Autodesk Inventor part; units mm, degrees
ref_plane "Work Plane1" through (0, 0, 0) normal (0, 0, 1) x (1, 0, 0)
ref_plane "Work Plane2" through (-10.1976, -10.1976, 2) normal (0, 0, 1) x (0.910504, -0.4135003, 0)
ref_plane "YZ Plane" through (0, 0, 0) normal (1, 0, 0) x (0, 1, 0)
ref_plane "Work Plane1" through (0, 0, 0) normal (0, 0, 1) x (1, 0, 0)
sketch "Sketch1" plane through (0, 0, 0) normal (0, 0, 1) x (1, 0, 0)
  circle A0 centre (0, 0) radius 12.5
  circle A1 centre (0, -18) radius 2
  circle A2 centre (0, 18) radius 2
  circle A3 centre (-18, 0) radius 2
  circle A4 centre (18, 0) radius 2
  circle A5 centre (11.3137, 11.3137) radius 1.6
  circle A6 centre (-11.3137, -11.3137) radius 1.6
  circle A7 centre (-11.3137, 11.3137) radius 1.6
  circle A8 centre (11.3137, -11.3137) radius 1.6
  circle A9 centre (0, 0) radius 20.7
  circle A10 centre (-11.3137, 11.3137) radius 1.2295
  circle A11 centre (0, 18) radius 1.621
  circle A12 centre (11.3137, 11.3137) radius 1.2295
  circle A13 centre (18, 0) radius 1.621
  circle A14 centre (11.3137, -11.3137) radius 1.2295
  circle A15 centre (-11.3137, -11.3137) radius 1.2295
  circle A16 centre (0, -18) radius 1.621
  circle A17 centre (-18, 0) radius 1.621
ref_plane "Work Plane2" through (-10.1976, -10.1976, 2) normal (0, 0, 1) x (0.910504, -0.4135003, 0)
extrude "Extrusion1" add sketch "Sketch1" along normal up to surface (2 mm away) contours A1 | A2 | A3 | A4 | A5 | A6 | A7 | A8 | A9
properties part number "gearboxspacer 2 mm"
Part model, mm, in its own coordinate system. Coordinates: 2 decimals unless noted, no trailing zeros. Order: outer loops, then holes, each group sorted by start corner. A loop starts at its lowest first (then second) coordinate and runs counter-clockwise, first axis right, second up. Notation, with made-up numbers: (-2, 82.5) - (10, 82.5) arc R5 cw to (10, 86.5) - close; hole circle Ø10 at (-38.75, 81). An arc over 180 degrees is marked (long way). Return JSON: item names as keys, results as strings. Group by question number.
Item 1: Pull direction X, two halves, no side cores. Call faces 1 (the face through (-16.427, 12.596, 0.986)), 2 (the face through (9, -9, 0)), 3 (the face through (-12.22, -12.145, 0.986)): pulls with the +X half, pulls with the -X half, needs draft (parallel to the pull), parting line crosses it, or undercut.
Item 2: Cut at B-B (y = 9). List the corners of the cut face in (x, z), plus the area to 3 significant figures.
Item 3: Drill centre lines: probe 1 along Y at (x, z) = (0, 1.3); probe 2 along Y at (x, z) = (-11, 0.8); probe 3 along X at (y, z) = (-1, 1.45). Where is each one in solid material? Low to high. Write a range as from..to.
Item 4: Cut at C-C (z = 0.4). State how many separate pieces and enclosed holes the cut face has, plus the area to 3 significant figures.
Item 5: Cut at A-A (x = 0). List the corners of the cut face in (y, z), plus the area to 3 significant figures.
Item 6: Cut at D-D (x = -18). List the corners of the cut face in (y, z).
Item 7: Pin check, flat tips, straight feed: pin 1 (1 mm diameter, centred on y = 2.5, z = 1.5, fed in from +X); pin 2 (1 mm diameter, centred on y = -1, z = 1.5, fed in from -X). Stop position of each tip, or through.
Check values:
{
 "1": {"face 1": "parting line crosses it", "face 2": "needs draft", "face 3": "undercut"},
 "2": {"outline": "(-18.64, 0) - (-8.67, 0) - (-8.67, 2) - (-18.64, 2) - close; (8.67, 0) - (18.64, 0) - (18.64, 2) - (8.67, 2) - close", "area": "39.9 mm2"},
 "3": {"probe 1": "y = -20.7..-19.62, -16.38..-12.5, 12.5..16.38, 19.62..20.7", "probe 2": "y = -17.54..-12.5, -10.12..-5.94, 5.94..10.12, 12.5..17.54", "probe 3": "x = -20.68..-19.28, -16.72..-12.46, 12.46..16.72, 19.28..20.68"},
 "4": {"separate pieces": "1", "enclosed holes": "9", "area": "803 mm2"},
 "5": {"outline": "(-20.7, 0) - (-19.62, 0) - (-19.62, 2) - (-20.7, 2) - close; (-16.38, 0) - (-12.5, 0) - (-12.5, 2) - (-16.38, 2) - close; (12.5, 0) - (16.38, 0) - (16.38, 2) - (12.5, 2) - close; (19.62, 0) - (20.7, 0) - (20.7, 2) - (19.62, 2) - close", "area": "19.8 mm2"},
 "6": {"outline": "(-10.22, 0) - (-1.62, 0) - (-1.62, 2) - (-10.22, 2) - close; (1.62, 0) - (10.22, 0) - (10.22, 2) - (1.62, 2) - close"},
 "7": {"pin 1": "stops at x = 20.6", "pin 2": "stops at x = -20.69"}
}
